For this review, take the finished solid that the model builds, in its own axes (mm). Coordinates: 2 decimals unless noted, no trailing zeros. Loops run counter-clockwise (first coordinate to the right, second up) from the corner with the lowest first, then second, coordinate; pieces in that order, holes last.
1. To check wall thickness, follow probe 1 along Y at (x, z) = (32, 1366.5); probe 2 along X at (y, z) = (3, 1100); probe 3 along Y at (x, z) = (35, 186). State the ranges of each line that lie inside material, in increasing order.
2. Clearance check with flat-ended pins moving along their axes: P1, Ø4, axis at y = 14, z = 757.5, coming from the +X side; P2, Ø6, axis at y = 8.5, z = 202.5, coming from the +X side; P3, Ø1.5, axis at x = 56.5, y = 6.5, coming from the -Z side. State where each tip first meets the part, or that it passes through.
3. Take a section at A-A, the plane z = 1243. State the section outline as (x, y) points.
4. Take a section at B-B, the plane y = 8. State the section outline as (x, z) points, then the cut area to 3 significant figures.
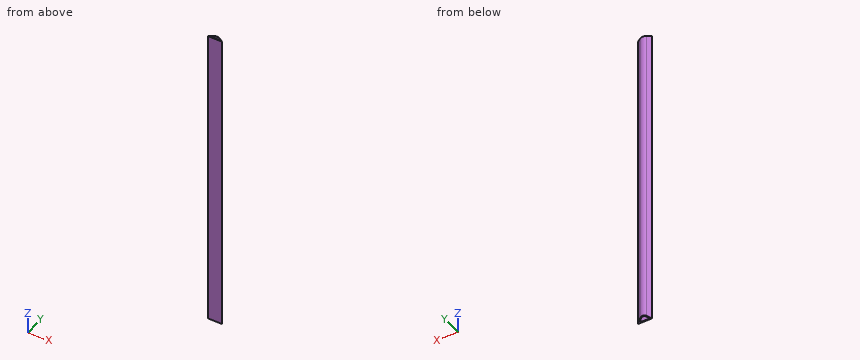
```python
from build123d import *

# Parameters (mm, degrees)
BOSS_EXTRUDE1_DEPTH = 1498.6
CUT_EXTRUDE1_DEPTH  = 69.58


with BuildPart() as part:
    # Sketch2 → Boss-Extrude1 (new body)
    with BuildSketch(Plane.XY):
        with BuildLine():
            Line((0, 0), (68.58, 0))
            Line((68.58, 0), (49.587320143, 13.03542143))
            ThreePointArc((49.587320143, 13.03542143), (34.29, 17.78), (18.992679857, 13.03542143))
            Line((18.992679857, 13.03542143), (0, 0))
        make_face()
        with BuildLine():
            Line((10.997802271, 4.46752515), (8.189387654, 2.54))
            Line((8.189387654, 2.54), (9.965035751, 2.54))
            ThreePointArc((9.965035751, 2.54), (10.461920618, 3.514209799), (10.997802271, 4.46752515))
        make_face(mode=Mode.SUBTRACT)
        with BuildLine():
            Line((57.582197729, 4.46752515), (60.390612346, 2.54))
            Line((60.390612346, 2.54), (58.614964249, 2.54))
            ThreePointArc((58.614964249, 2.54), (58.118079382, 3.514209799), (57.582197729, 4.46752515))
        make_face(mode=Mode.SUBTRACT)
        with BuildLine():
            Line((12.82308193, 2.54), (55.75691807, 2.54))
            ThreePointArc((55.75691807, 2.54), (34.29, 15.24), (12.82308193, 2.54))
        make_face(mode=Mode.SUBTRACT)
    extrude(amount=BOSS_EXTRUDE1_DEPTH)

    # Sketch3 → Cut-Extrude1 (cut, through all)
    with BuildSketch(Plane(origin=(0, 0, 0), x_dir=(0, 0, -1), z_dir=(1, 0, 0))):
        Polygon((-17.78, 17.78), (0, 0), (0, 17.78), align=None)
    extrude(amount=CUT_EXTRUDE1_DEPTH, mode=Mode.SUBTRACT)


solid = part.part
```
Results list:
1. probe 1: y = 0 to 2.54, 15.13 to 17.68
1. probe 2: x = 4.37 to 8.86, 10.19 to 13.08, 55.5 to 58.39, 59.72 to 64.21
1. probe 3: y = 0 to 2.54, 15.23 to 17.77
2. P1: stops at x = 51.1
2. P2: stops at x = 60.57
2. P3: stops at z = 5.75
3. outline: (0, 0) - (68.58, 0) - (49.59, 13.04) arc R27.03 ccw to (18.99, 13.04) - close; hole (8.19, 2.54) - (9.97, 2.54) arc R27.03 cw to (11, 4.47) - close; hole (12.82, 2.54) - (55.76, 2.54) arc R24.49 ccw to start; hole (57.58, 4.47) arc R27.03 cw to (58.61, 2.54) - (60.39, 2.54) - close
4. outline: (11.66, 8) - (16.9, 8) - (16.9, 1498.6) - (11.66, 1498.6) - close; (51.68, 8) - (56.92, 8) - (56.92, 1498.6) - (51.68, 1498.6) - close
4. area: 15,600 mm2
